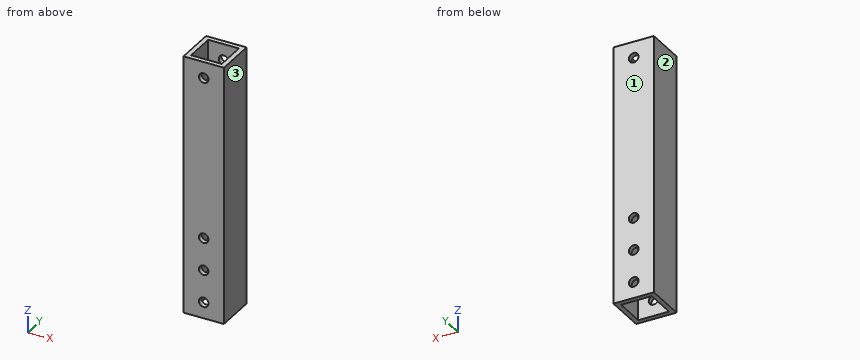
from build123d import *

# Parameters (mm, degrees)
SKETCH1_W           = 25
SKETCH1_H           = 25
SKETCH1_W_2         = 19
SKETCH1_H_2         = 19
BOSS_EXTRUDE1_DEPTH = 160
SKETCH2_R           = 3
CUT_EXTRUDE1_DEPTH  = 26


with BuildPart() as part:
    # Sketch1 → Boss-Extrude1 (new body)
    with BuildSketch(Plane.XY):
        with Locations((12.5, 12.5)):
            Rectangle(SKETCH1_W, SKETCH1_H)
        with Locations((12.5, 12.5)):
            Rectangle(SKETCH1_W_2, SKETCH1_H_2, mode=Mode.SUBTRACT)
    extrude(amount=BOSS_EXTRUDE1_DEPTH)

    # Sketch2 → Cut-Extrude1 (cut, through all)
    with BuildSketch(Plane.XZ):
        with Locations((12.5, 10)):
            Circle(SKETCH2_R)
        with Locations((12.5, 30)):
            Circle(SKETCH2_R)
        with Locations((12.5, 50)):
            Circle(SKETCH2_R)
        with Locations((12.5, 150)):
            Circle(SKETCH2_R)
    extrude(amount=-CUT_EXTRUDE1_DEPTH, mode=Mode.SUBTRACT)


solid = part.part
Geometry: final body of the model. Coordinates: model frame, mm. Face numbers are marked on the shaded views. Give positions to 0.01 mm unless a question says otherwise; leave off trailing zeros. Write each loop counter-clockwise with the first axis right and the second up, starting at its lowest first coordinate (ties: lowest second). Pieces come first, ordered by that corner, then holes. Notation, with made-up numbers: M 43,-3.75 L 55,-3.75 A21 ccw 55,23.25 Z; hole C 36,68 d3. An arc over 180 degrees is marked long. Answer in a Markdown table with one row per item. Add a question column.
(1) Section A-A on z = 30. Return loops of the section in (x, y), and give its area (3 significant figures).
(2) Section B-B on x = 19.25. Return loops of the section in (y, z), and give its area (3 significant figures).
(3) Section D-D on x = 12.5. State how many separate pieces and enclosed holes the cut face has, and give its area (3 significant figures).
(4) Ray query, line 1 (Z direction, x = 12.5, y = 1.3); line 2 (X direction, y = 20.75, z = 75.5). Return the intervals inside material, ascending.
(5) Mould query, pull axis X, two halves, no side actions, for the marked faces 1, 2 and 3. Classes: +X half, -X half, draft (parallel to the pull), parting line (faces both ways), or undercut.
Result set:
| question | item | result |
|---|---|---|
| 1 | outline | M 0,0 L 9.5,0 L 9.5,3 L 3,3 L 3,22 L 9.5,22 L 9.5,25 L 0,25 Z; M 15.5,0 L 25,0 L 25,25 L 15.5,25 L 15.5,22 L 22,22 L 22,3 L 15.5,3 Z |
| 1 | area | 228 mm^2 |
| 2 | outline | M 0,0 L 3,0 L 3,160 L 0,160 Z; M 22,0 L 25,0 L 25,160 L 22,160 Z |
| 2 | area | 960 mm^2 |
| 3 | separate pieces | 10 |
| 3 | enclosed holes | 0 |
| 3 | area | 816 mm^2 |
| 4 | line 1 | z = 0 to 7, 13 to 27, 33 to 47, 53 to 147, 153 to 160 |
| 4 | line 2 | x = 0 to 3, 22 to 25 |
| 5 | face 1 | draft |
| 5 | face 2 | -X half |
| 5 | face 3 | +X half |
